```python
from build123d import *

# Parameters (mm, degrees)
F0_R     = 31.75
F1_DEPTH = 3.175
F2_R     = 27.7495
F3_DEPTH = 18.034
F5_DEPTH = 25.4
F6_R     = 1.5875


with BuildPart() as f1:
    # F0 (on Top) → F1 (new body)
    with BuildSketch(Plane.XY):
        Circle(F0_R)
    extrude(amount=F1_DEPTH)

    # F2 (on face) → F3 (join)
    with BuildSketch(Plane.XY.offset(3.175)):
        Circle(F2_R)
    extrude(amount=F3_DEPTH)

    # F4 (on face) → F5 (cut)
    with BuildSketch(Plane(origin=(0, 0, 0), x_dir=(1, 0, 0), z_dir=(0, 0, -1))):
        with BuildLine():
            ThreePointArc((31.75, 0), (31.627275, 2.788905), (31.260048, 5.55625))
            Line((31.260048, 5.55625), (21.7424, 5.55625))
            ThreePointArc((21.7424, 5.55625), (16.18615, 0), (21.7424, -5.55625))
            Line((21.7424, -5.55625), (31.260048, -5.55625))
            ThreePointArc((31.260048, -5.55625), (31.627275, -2.788905), (31.75, 0))
        make_face()
    extrude(amount=-F5_DEPTH, mode=Mode.SUBTRACT)

    # F6
    f6_edges = [f1.edges().sort_by_distance(p)[0] for p in [
        (-31.75, 0, 0),
        (26.501224, -5.55625, 0),
        (16.18615, 0, 0),
        (26.501224, 5.55625, 0),
    ]]
    fillet(f6_edges, radius=F6_R)


solid = f1.part
```
CAD build for the part. Positions are in the model's coordinates, mm. A direction names the side the tool comes from. Round coordinates to 2 decimals unless told otherwise and drop trailing zeros. Order: outer loops, then holes, each group sorted by start corner. A loop starts at its lowest first (then second) coordinate and runs counter-clockwise, first axis right, second up. Notation, with made-up numbers: (77, -40) -> (109, -40) arc R26 ccw to (109, -9) -> close; hole circle Ø2 at (75.5, -19.75). An arc over 180 degrees is marked (long way). One line per question, with ' | ' between items.
Q1. Two-plate mould, pull along Y, no slides. Class faces 4 (the flat face through (-28, 0, 3.175)), 5 (the flat face through (24, 5.556, 11)), 6 (the cylindrical face through (-31.723, 1.318, 2.37)): released by +Y, released by -Y, zero draft, split by the parting line, or undercut.
Completed:
face 4: zero draft | face 5: undercut | face 6: split by the parting line
Q2. Which spindle directions (+Z, -Z, +X, -X, +Y, -Y) get a long thin tool onto all of the face, cutting with end or side? Do faces 1 (the flat face through (24, -5.556, 11)), 2 (the cylindrical face through (26.568, 6.034, 0.453)), 3 (the cylindrical face through (-27.726, 1.142, 12.066)). Say none if no direction does.
Completed:
face 1: +Z, -Z, +X | face 2: -Z, +X | face 3: +Z
Q3. Slice it at C-C (z = 18.25). Write the cut outline in (x, y), then the cut area to 3 significant figures.
Completed:
outline: (21.74, -5.56) arc R5.56 cw to (21.74, 5.56) -> (27.19, 5.56) arc R27.75 ccw (long way) to (27.19, -5.56) -> close | area: 2,310 mm^2
Q4. Drop flat-ended pins along their axis: pin 1 (5 mm diameter, centred on y = 25, z = 16.5, fed in from +X); pin 2 (12 mm diameter, centred on x = 3.5, z = 10.5, fed in from -Y); pin 3 (6 mm diameter, centred on x = 9, z = 15, fed in from -Y). Give the stop position or say it passes through.
Completed:
pin 1: stops at x = 16.24 | pin 2: stops at y = -27.75 | pin 3: stops at y = -27.09
Q5. Probe probe 1 along Z at (x, y) = (-22.5, -17) (3 decimals); probe 2 along Y at (x, z) = (27, 2.5); probe 3 along Y at (x, z) = (26, 3). List the from-to ranges inside material, lowest first.
Completed:
probe 1: z = 0 to 3.175 | probe 2: y = -16.71 to -5.56, 5.56 to 16.71 | probe 3: y = -18.22 to -5.56, 5.56 to 18.22
